from build123d import *

# Parameters (mm, degrees)
SKETCH1_W           = 134.62
SKETCH1_H           = 78.74
BOSS_EXTRUDE1_DEPTH = 2.286
SKETCH2_W           = 129.54
SKETCH2_H           = 68.58
BOSS_EXTRUDE2_DEPTH = 5.334
SKETCH3_W           = 139.7
SKETCH3_H           = 88.9
BOSS_EXTRUDE3_DEPTH = 5.08


with BuildPart() as part:
    # Sketch1 → Boss-Extrude1 (new body)
    with BuildSketch(Plane(origin=(0, 0, 0), x_dir=(1, 0, 0), z_dir=(0, 1, 0))):
        with Locations((72.236796638, -12.067156206)):
            Rectangle(SKETCH1_W, SKETCH1_H)
    extrude(amount=BOSS_EXTRUDE1_DEPTH)

    # Sketch2 → Boss-Extrude2 (add)
    with BuildSketch(Plane(origin=(0, 2.286, 0), x_dir=(1, 0, 0), z_dir=(0, 1, 0))):
        with Locations((69.696796638, -12.067156206)):
            Rectangle(SKETCH2_W, SKETCH2_H)
    extrude(amount=BOSS_EXTRUDE2_DEPTH)

    # Sketch3 → Boss-Extrude3 (add)
    with BuildSketch(Plane(origin=(0, 7.62, 0), x_dir=(1, 0, 0), z_dir=(0, 1, 0))):
        with Locations((74.776796638, -12.067156206)):
            Rectangle(SKETCH3_W, SKETCH3_H)
    extrude(amount=BOSS_EXTRUDE3_DEPTH)


solid = part.part
Could you check a few things on this model? Use its own coordinates, in mm. A direction names the side the tool comes from. Coordinates: 2 decimals unless noted, no trailing zeros. Loops run counter-clockwise (first coordinate to the right, second up) from the corner with the lowest first, then second, coordinate; pieces in that order, holes last.
1. Imagine slicing it at B-B (z = 5). Please give me the cut outline in (x, y), and give its area (3 significant figures).
2. I need wall thicknesses on L1, parallel to Y at x = 135, z = -15.5; L2, parallel to X at y = 5.5, z = -8.5; L3, parallel to X at y = 0.5, z = -10.5. Which ranges of each line are inside material? Lowest first, please.
3. Imagine slicing it at C-C (y = 4.25). Please give me the cut outline in (x, z), and give its area (3 significant figures).
4. We'd pull the mould along Y, two halves only. Please class faces 5 (the face through (74, 10, 56.517)), 6 (the face through (82, 2.286, 47)), 7 (the face through (74, 12.7, 11)): released by +Y, released by -Y, zero draft, split by the parting line, or undercut.
5. Imagine slicing it at A-A (x = 80). Please give me the cut outline in (y, z).
6. For faces 1 (the face through (134.467, 5, 13)), 2 (the face through (69, 5, 46.357)), 3 (the face through (90, 7.62, 48)), 4 (the face through (69, 5, -22.223)), which set-ups out of +Z, -Z, +X, -X, +Y, -Y let a thin tool reach every point of the face, with its end or its side?
7. For P1, Ø1.5, axis at x = 77, y = 6.5, coming from the +Z side; P2, Ø1.6, axis at y = 6, z = 9, coming from the +X side; P3, Ø1.1, axis at y = 1, z = 16, coming from the +X side, each with a flat end and sliding along its axis, tell me the tip position at first contact or that it passes through.
Computed values:
1. outline: (4.93, 0) - (139.55, 0) - (139.55, 2.29) - (134.47, 2.29) - (134.47, 7.62) - (144.63, 7.62) - (144.63, 12.7) - (4.93, 12.7) - close
1. area: 1,710 mm2
2. L1: y = 0 to 2.29, 7.62 to 12.7
2. L2: x = 4.93 to 134.47
2. L3: x = 4.93 to 139.55
3. outline: (4.93, -22.22) - (134.47, -22.22) - (134.47, 46.36) - (4.93, 46.36) - close
3. area: 8,880 mm2
4. face 5: zero draft
4. face 6: undercut
4. face 7: released by +Y
5. outline: (0, -27.3) - (2.29, -27.3) - (2.29, -22.22) - (7.62, -22.22) - (7.62, -32.38) - (12.7, -32.38) - (12.7, 56.52) - (7.62, 56.52) - (7.62, 46.36) - (2.29, 46.36) - (2.29, 51.44) - (0, 51.44) - close
6. face 1: +Z, -Z, +X
6. face 2: +Z, +X, -X
6. face 3: +X
6. face 4: -Z, +X, -X
7. P1: stops at z = 46.36
7. P2: stops at x = 134.47
7. P3: stops at x = 139.55
